from build123d import *

# Parameters (mm, degrees)
ESQUISSE1_R        = 25
BOSS_EXTRU_1_DEPTH = 10
ESQUISSE2_R        = 15
BOSS_EXTRU_2_DEPTH = 3
ESQUISSE3_R        = 4
BOSS_EXTRU_3_DEPTH = 6
CONG_1_R           = 10
CONG_2_R           = 1
CONG_3_R           = 10


# Some blends are built 0.0001 mm under size
with BuildPart() as part:
    # Esquisse1 → Boss.-Extru.1 (new body)
    with BuildSketch(Plane.XY):
        Circle(ESQUISSE1_R)
    extrude(amount=BOSS_EXTRU_1_DEPTH)

    # Esquisse2 → Boss.-Extru.2 (add)
    with BuildSketch(Plane.XY.offset(10)):
        Circle(ESQUISSE2_R)
    extrude(amount=BOSS_EXTRU_2_DEPTH)

    # Esquisse3 → Boss.-Extru.3 (add)
    with BuildSketch(Plane.XY.offset(13)):
        Circle(ESQUISSE3_R)
    extrude(amount=BOSS_EXTRU_3_DEPTH)

    # Congé1
    # the kernel refuses this fillet: 10 mm, written as the material it takes off along each edge
    with BuildSketch(Plane(origin=(0, 0, 13), x_dir=(1, 0, 0), z_dir=(0, -1, 0))) as cong_1_piece_1:
        with BuildLine():
            CenterArc((7.858571571, -10), CONG_1_R, 44.427004001, 45.572995999)
            Line((7.858571571, 0), (7.858571571, 0.2))
            Line((7.858571571, 0.2), (15, 0.2))
            Line((15, 0.2), (15.2, 0))
            ThreePointArc((15.2, 0), (15.2, -1.5), (15.142828569, -2.86))
            Line((15.142828569, -2.86), (15, -3))
        make_face()
    revolve(axis=Axis((0, 0, 13), (0, 0, 1)), mode=Mode.SUBTRACT)

    # Congé2
    cong_2_edges = [part.edges().sort_by_distance(p)[0] for p in [
        (-4, 0, 19),
    ]]
    fillet(cong_2_edges, radius=CONG_2_R)

    # Congé3
    cong_3_edges = [part.edges().sort_by_distance(p)[0] for p in [
        (-25, 0, 10),
    ]]
    fillet(cong_3_edges, radius=CONG_3_R - 0.0001)  # a hair under: the kernel refuses the full size


solid = part.part
Verification items for the finished model (mm, model axes). A direction names the side the tool comes from. Coordinates: 2 decimals unless noted, no trailing zeros. Order: outer loops, then holes, each group sorted by start corner. A loop starts at its lowest first (then second) coordinate and runs counter-clockwise, first axis right, second up.
1. Scan lines: line 1 (Z direction, x = 0.5, y = -15.5); line 2 (Z direction, x = 4.5, y = -9); line 3 (X direction, y = -2, z = 2.5). Record each from-to range of solid material in increasing order.
Results found:
line 1: z = 0 to 9.99
line 2: z = 0 to 12.75
line 3: x = -24.6 to 24.6
2. Sectioned sample at A-A, the plane z = 16. Record the cut outline in (x, y), and give its area (3 significant figures).
Results found:
outline: circle Ø8 at (0, 0)
area: 50.3 mm2
3. Set-up check for faces 1 (the face through (-0.867, -3.905, 15.465)), 2 (the face through (0, 0, 0)): record each of +Z, -Z, +X, -X, +Y, -Y from which the full face is reachable in a straight line by a thin tool's end or side.
Results found:
face 1: +Z
face 2: -Z, +X, -X, +Y, -Y
4. Go/stop test with flat-tipped pins: pin 1 Ø6 at (y, z) = (6, 6) entering from +X; pin 2 Ø3 at (y, z) = (-5.5, 13.5) entering from -X; pin 3 Ø3 at (x, z) = (-16.5, 6) entering from +Y. Record where each tip stops, or that it passes through.
Results found:
pin 1: stops at x = 23.99
pin 2: stops at x = -10.99
pin 3: stops at y = 17.98
5. Sectioned sample at B-B, the plane z = 2.75. Record the cut outline in (x, y).
Results found:
outline: circle Ø49.23 at (0, 0)
